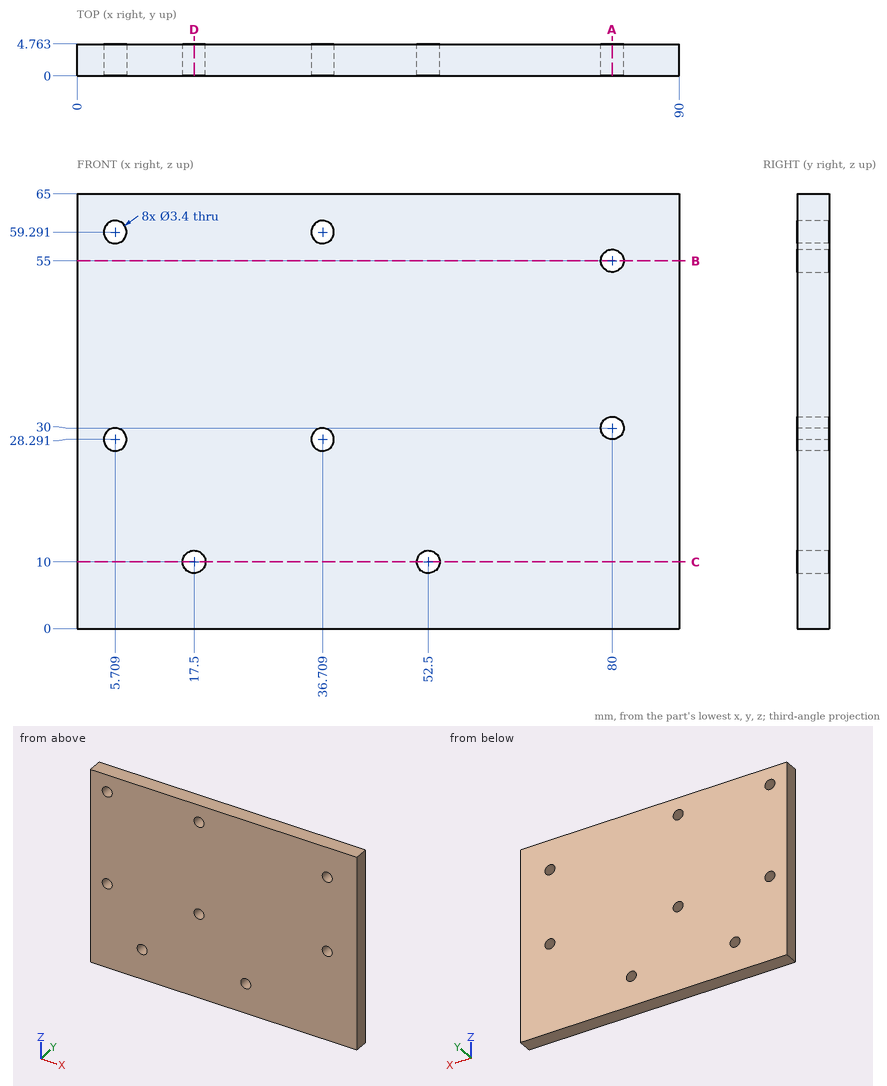
The figure shows three views and two pictorial views of one solid part (mm, origin at its lowest corner). Answer the questions. Give positions to 0.01 mm unless a question says otherwise; leave off trailing zeros. Loops run counter-clockwise (first coordinate to the right, second up) from the corner with the lowest first, then second, coordinate; pieces in that order, holes last. Notation, with made-up numbers: (58.25, 25.25) -> (69.25, 25.25) arc R17 ccw to (69.25, 44.25) -> close; hole circle Ø6 at (42, -7.5). An arc over 180 degrees is marked (long way). Use a Markdown table: item, result. Add a question column.
1. Section D-D on x = 17.5 is taken. Determine the outline of the cut face in (y, z).
2. Flat-ended cylindrical pins translate along their axes: pin 1 Ø3 at (x, z) = (36.709, 59.291) entering from +Y; pin 2 Ø4.5 at (x, z) = (80, 30) entering from -Y. Find the tip coordinate at first contact, or state that the pin passes through.
3. Section B-B on z = 55 is taken. Determine the outline of the cut face in (x, y).
4. Section C-C on z = 10 is taken. Determine the outline of the cut face in (x, y).
5. Section A-A on x = 80 is taken. Determine the outline of the cut face in (y, z), and give its area (3 significant figures).
6. Find the intervals of material crossed by probe 1 along Z at (x, y) = (80, 2.1); probe 2 along X at (y, z) = (0.3, 55); probe 3 along X at (y, z) = (1.15, 60) (1 decimal), in increasing order.
Results below:
| question | item | result |
|---|---|---|
| 1 | outline | (0, 0) -> (4.76, 0) -> (4.76, 8.3) -> (0, 8.3) -> close; (0, 11.7) -> (4.76, 11.7) -> (4.76, 65) -> (0, 65) -> close |
| 2 | pin 1 | passes through |
| 2 | pin 2 | stops at y = 0 |
| 3 | outline | (0, 0) -> (78.3, 0) -> (78.3, 4.76) -> (0, 4.76) -> close; (81.7, 0) -> (90, 0) -> (90, 4.76) -> (81.7, 4.76) -> close |
| 4 | outline | (0, 0) -> (15.8, 0) -> (15.8, 4.76) -> (0, 4.76) -> close; (19.2, 0) -> (50.8, 0) -> (50.8, 4.76) -> (19.2, 4.76) -> close; (54.2, 0) -> (90, 0) -> (90, 4.76) -> (54.2, 4.76) -> close |
| 5 | outline | (0, 0) -> (4.76, 0) -> (4.76, 28.3) -> (0, 28.3) -> close; (0, 31.7) -> (4.76, 31.7) -> (4.76, 53.3) -> (0, 53.3) -> close; (0, 56.7) -> (4.76, 56.7) -> (4.76, 65) -> (0, 65) -> close |
| 5 | area | 277 mm^2 |
| 6 | probe 1 | z = 0 to 28.3, 31.7 to 53.3, 56.7 to 65 |
| 6 | probe 2 | x = 0 to 78.3, 81.7 to 90 |
| 6 | probe 3 | x = 0 to 4.2, 7.3 to 35.2, 38.3 to 90 |
